Verification items for the finished model (mm, model axes). Face numbers are marked on the shaded views. A direction names the side the tool comes from. Coordinates: 2 decimals unless noted, no trailing zeros. Write each loop counter-clockwise with the first axis right and the second up, starting at its lowest first coordinate (ties: lowest second). Pieces come first, ordered by that corner, then holes. Notation, with made-up numbers: (87, 5) -> (135, 5) arc R31 ccw to (135, 43) -> close; hole circle Ø1 at (8.25, 12). An arc over 180 degrees is marked (long way). Answer in a Markdown table with one row per item.
```python
from build123d import *

# Parameters (mm, degrees)
F0_W     = 98.3961671591
F0_H     = 55.4385446012
F1_DEPTH = 101.6
F2_R     = 25.4
F3_DEPTH = 25.4
F5_DEPTH = 25.399999693
F6_R     = 6.6402223844
F7_DEPTH = 25


with BuildPart() as f1:
    # F0 (on Front) → F1 (new body)
    with BuildSketch(Plane.XZ):
        with Locations((49.1980835795, 27.7192723006)):
            Rectangle(F0_W, F0_H)
    extrude(amount=F1_DEPTH)

    # F2 (on face) → F3 (cut)
    with BuildSketch(Plane.XY.offset(55.4385446012)):
        with Locations((50.8, -50.8)):
            Circle(F2_R)
    extrude(amount=-F3_DEPTH, mode=Mode.SUBTRACT)

    # F4 (on face) → F5 (join)
    with BuildSketch(Plane.XY.offset(55.4385446012)):
        Polygon((49.1980835795, -101.6), (0, -50.8), (0, -101.6), align=None)
    extrude(amount=F5_DEPTH)

    # F6 (on face) → F7 (cut)
    with BuildSketch(Plane(origin=(-25.386966873, -24.5864196466, 0), x_dir=(-0.695690045, 0.7183420921, 0), z_dir=(0.7183420921, 0.695690045, 0))):
        with Locations((-71.5789571404, 69.76454705)):
            Circle(F6_R)
    extrude(amount=-F7_DEPTH, mode=Mode.SUBTRACT)


solid = f1.part
```
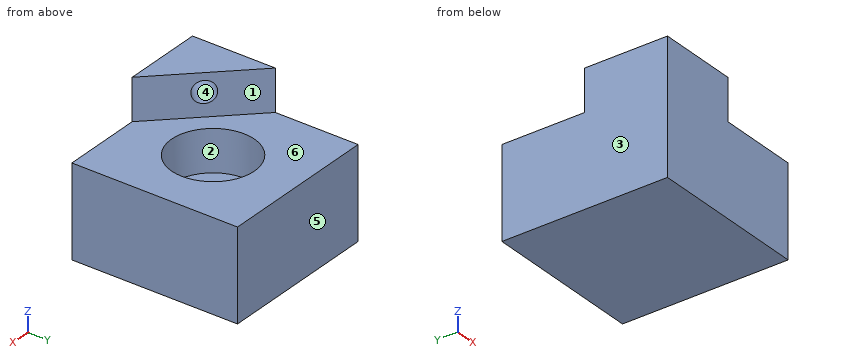
1. Section check A-A, the plane x = 50.8. Record the boundary of the cut face in (y, z), plus the area to 3 significant figures.
Geometry says:
| item | result |
|---|---|
| outline | (-101.6, 0) -> (0, 0) -> (0, 55.44) -> (-25.4, 55.44) -> (-25.4, 30.04) -> (-76.2, 30.04) -> (-76.2, 55.44) -> (-101.6, 55.44) -> close |
| area | 4,340 mm^2 |
2. Section check C-C, the plane y = -34.5. Record the boundary of the cut face in (x, z), plus the area to 3 significant figures.
Geometry says:
| item | result |
|---|---|
| outline | (0, 0) -> (98.4, 0) -> (98.4, 55.44) -> (70.28, 55.44) -> (70.28, 30.04) -> (31.32, 30.04) -> (31.32, 55.44) -> (0, 55.44) -> close |
| area | 4,470 mm^2 |
3. Thickness scan on line 1 (Z direction, x = 88, y = -67); line 2 (Y direction, x = 50, z = 46); line 3 (Z direction, x = 58, y = -52). Record the ranges inside material, lowest first. Write a range as from..to.
Geometry says:
| item | result |
|---|---|
| line 1 | 0..55.44 |
| line 2 | -101.6..-76.19, -25.41..0 |
| line 3 | 0..30.04 |
4. Tool access check on the marked faces 5 and 6. Record the directions out of +Z, -Z, +X, -X, +Y, -Y that give a thin tool (end or side, any length) a straight path to the whole face; none if there is none.
Geometry says:
| item | result |
|---|---|
| face 5 | +Z, -Z, +X, -X, +Y |
| face 6 | +Z, +X, +Y |
5. Mould release check, pull along X, two halves, no side actions. Record for the marked faces 1, 2, 3 and 4: released by +X, released by -X, zero draft, split by the parting line, or undercut.
Geometry says:
| item | result |
|---|---|
| face 1 | released by +X |
| face 2 | undercut |
| face 3 | released by -X |
| face 4 | undercut |
6. Section check D-D, the plane z = 65. Record the boundary of the cut face in (x, y).
Geometry says:
| item | result |
|---|---|
| outline | (0, -101.6) -> (49.2, -101.6) -> (27.63, -79.33) -> (9.67, -96.72) -> (3.23, -90.07) -> (21.19, -72.68) -> (0, -50.8) -> close |
7. Section check B-B, the plane z = 36.5. Record the boundary of the cut face in (x, y), plus the area to 3 significant figures.
Geometry says:
| item | result |
|---|---|
| outline | (0, -101.6) -> (98.4, -101.6) -> (98.4, 0) -> (0, 0) -> close; hole circle Ø50.8 at (50.8, -50.8) |
| area | 7,970 mm^2 |
8. Depth check by flat-ended pin: P1, Ø3, axis at x = 72, y = -30.5, coming from the -Z side; P2, Ø1, axis at x = 67.5, y = -36.5, coming from the +Z side; P3, Ø8, axis at x = 17.5, y = -24, coming from the +Z side. Enter the tip coordinate at first touch or a pass-through.
Geometry says:
| item | result |
|---|---|
| P1 | z = 0 |
| P2 | z = 30.04 |
| P3 | z = 55.44 |
